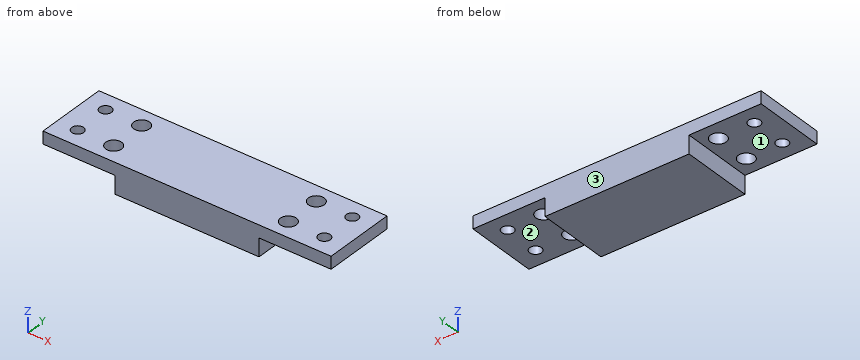
from build123d import *

# Parameters (mm, degrees)
SKETCH_1_W          = 60
SKETCH_1_H          = 20
EXTRUDE_1_DEPTH     = 3.45
SKETCH_2_W          = 40
SKETCH_2_H          = 20
EXTRUDE_2_DEPTH     = 5
SKETCH_4_W          = 80
SKETCH_4_H          = 20
EXTRUDE_3_DEPTH     = 3.45
SKETCH_7_R          = 2.2
SKETCH_7_R_2        = 1.65
CUT_EXTRUDE_1_DEPTH = 3.45


with BuildPart() as part:
    # 草图1 → 凸台-拉伸1 (new body)
    with BuildSketch(Plane.XY):
        with Locations((30, 10)):
            Rectangle(SKETCH_1_W, SKETCH_1_H)
    extrude(amount=EXTRUDE_1_DEPTH)

    # 草图2 → 凸台-拉伸2 (add)
    with BuildSketch(Plane(origin=(0, 0, 0), x_dir=(-1, 0, 0), z_dir=(0, 0, -1))):
        with Locations((-30, 10)):
            Rectangle(SKETCH_2_W, SKETCH_2_H)
    extrude(amount=EXTRUDE_2_DEPTH)

    # 草图4 → 凸台-拉伸3 (add)
    with BuildSketch(Plane(origin=(0, 0, 0), x_dir=(-1, 0, 0), z_dir=(0, 0, -1))):
        with Locations((-30, 10)):
            Rectangle(SKETCH_4_W, SKETCH_4_H)
    extrude(amount=-EXTRUDE_3_DEPTH)

    # 草图7 → 切除-拉伸1 (cut)
    with BuildSketch(Plane.XY.offset(3.45)):
        with Locations((5.75, 15.001516812)):
            Circle(SKETCH_7_R)
        with Locations((54.25, 15)):
            Circle(SKETCH_7_R)
        with Locations((54.25, 5)):
            Circle(SKETCH_7_R)
        with Locations((5.75, 5)):
            Circle(SKETCH_7_R)
        with Locations((-4.249999943, 15.000444876)):
            Circle(SKETCH_7_R_2)
        with Locations((-4.249999943, 5)):
            Circle(SKETCH_7_R_2)
        with Locations((64.25, 5)):
            Circle(SKETCH_7_R_2)
        with Locations((64.25, 15)):
            Circle(SKETCH_7_R_2)
    extrude(amount=-CUT_EXTRUDE_1_DEPTH, mode=Mode.SUBTRACT)


solid = part.part
Could you check a few things on this model? Use its own coordinates, in mm. Face numbers are marked on the shaded views. A direction names the side the tool comes from. Give positions to 0.01 mm unless a question says otherwise; leave off trailing zeros. Order: outer loops, then holes, each group sorted by start corner. A loop starts at its lowest first (then second) coordinate and runs counter-clockwise, first axis right, second up.
1. Which directions (+Z, -Z, +X, -X, +Y, -Y) give clear straight access to the entire face, cutting with the end or side of a thin tool? Please do the marked faces 1, 2 and 3.
Answers below:
face 1: -Z, -X, +Y, -Y
face 2: -Z, +X, +Y, -Y
face 3: +Z, -Z, +X, -X, +Y
2. Suppose I cut it at D-D (z = 2.25). State how many separate pieces and enclosed holes the cut face has, plus the area to 3 significant figures.
Answers below:
separate pieces: 1
enclosed holes: 8
area: 1,500 mm2
3. I need wall thicknesses on L1, parallel to Y at x = 64.25, z = 1.8; L2, parallel to Y at x = 5.75, z = 0.7; L3, parallel to Z at x = 9, y = 14.25. Which ranges of each line are inside material? Lowest first, please.
Answers below:
L1: y = 0 to 3.35, 6.65 to 13.35, 16.65 to 20
L2: y = 0 to 2.8, 7.2 to 12.8, 17.2 to 20
L3: z = 0 to 3.45
4. Suppose I cut it at B-B (x = 54.25). Write out the boundary of the cut face in (y, z), plus the area to 3 significant figures.
Answers below:
outline: (0, 0) - (2.8, 0) - (2.8, 3.45) - (0, 3.45) - close; (7.2, 0) - (12.8, 0) - (12.8, 3.45) - (7.2, 3.45) - close; (17.2, 0) - (20, 0) - (20, 3.45) - (17.2, 3.45) - close
area: 38.6 mm2
5. Suppose I cut it at C-C (y = 10). Write out the boundary of the cut face in (x, z), plus the area to 3 significant figures.
Answers below:
outline: (-10, 0) - (10, 0) - (10, -5) - (50, -5) - (50, 0) - (70, 0) - (70, 3.45) - (-10, 3.45) - close
area: 476 mm2
6. Suppose I cut it at A-A (y = 5). Write out the boundary of the cut face in (x, z), plus the area to 3 significant figures.
Answers below:
outline: (-10, 0) - (-5.9, 0) - (-5.9, 3.45) - (-10, 3.45) - close; (-2.6, 0) - (3.55, 0) - (3.55, 3.45) - (-2.6, 3.45) - close; (7.95, 0) - (10, 0) - (10, -5) - (50, -5) - (50, 0) - (52.05, 0) - (52.05, 3.45) - (7.95, 3.45) - close; (56.45, 0) - (62.6, 0) - (62.6, 3.45) - (56.45, 3.45) - close; (65.9, 0) - (70, 0) - (70, 3.45) - (65.9, 3.45) - close
area: 423 mm2
7. For pin 1 (1.5 mm diameter, centred on x = 7.5, y = 6, fed in from -Z), with a flat end and sliding along its axis, tell me the tip position at first contact or that it passes through.
Answers below:
pin 1: stops at z = 0
